Work out the finished part from the listing and answer in its coordinate system (mm). Face numbers are marked on the shaded views. A direction names the side the tool comes from. Give positions to 0.01 mm unless a question says otherwise; leave off trailing zeros. Loops run counter-clockwise (first coordinate to the right, second up) from the corner with the lowest first, then second, coordinate; pieces in that order, holes last. Notation, with made-up numbers: M 88,89.25 L 117,89.25 A18 ccw 117,119.25 Z; hole C -30.75,-39.75 d5. An arc over 180 degrees is marked long. Write item = value, one per line. Start each with the question number.
1. Section B-B on y = 84 is taken. Determine the outline of the cut face in (x, z).
2. Flat-ended cylindrical pins translate along their axes: pin 1 Ø2.5 at (x, z) = (20, 23) entering from -Y; pin 2 Ø2 at (x, z) = (17.5, 16) entering from +Y; pin 3 Ø1 at (x, z) = (4, 9) entering from +Y. Find the tip coordinate at first contact, or state that the pin passes through.
3. For the marked faces 1, 2 and 3, determine the directions among +Z, -Z, +X, -X, +Y, -Y from which every point of the face is accessible in a straight line to the end or side of a thin tool.
4. Section A-A on y = 0 is taken. Determine the outline of the cut face in (x, z) (3 decimals), plus the area to 3 significant figures.
5. Consider L1, parallel to Y at x = 33.35, z = 6; L2, parallel to X at y = -20.5, z = 17.25; L3, parallel to Y at x = 23.5, z = 14.75. Determine where each line is inside the solid, lowest interval first. Write a range as [from, to].
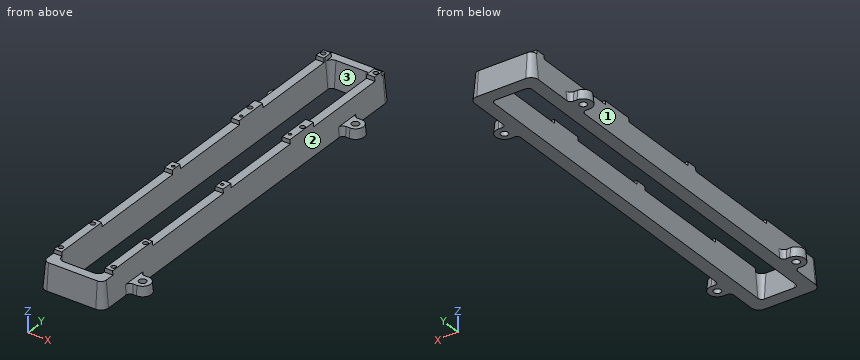
```python
from build123d import *

# Parameters (mm, degrees)
F1_DEPTH      = 25.4
F1_TAPER      = 5
F3_DEPTH      = 304.8010001
F3_DEPTH_BACK = 38.1010001
F4_W          = 70.425
F4_H          = 3.4
F4_W_2        = 84.225
F5_DEPTH      = 40.7760001
F5_DEPTH_BACK = 40.7760001
F6_W          = 73
F6_H          = 3.4
F7_DEPTH      = 40.7760001
F7_DEPTH_BACK = 40.7760001
F9_DEPTH      = 16.0010001
F10_R         = 3.1
F11_DEPTH     = 25.4010001
F12_R         = 2
F12_R_2       = 1.25
F13_DEPTH     = 11


with BuildPart() as f1:
    # F0 (on Top) → F1 (new body)
    with BuildSketch(Plane.XY):
        with BuildLine():
            Line((20.65, 304.8), (-20.65, 304.8))
            ThreePointArc((-20.65, 304.8), (-25.1401280605, 302.9401280605), (-27, 298.45))
            Line((-27, 298.45), (-27, 264.625))
            ThreePointArc((-27, 264.625), (-27.9372583002, 262.3622583002), (-30.2, 261.425))
            Line((-30.2, 261.425), (-33.35, 261.425))
            ThreePointArc((-33.35, 261.425), (-40.775, 254), (-33.35, 246.575))
            Line((-33.35, 246.575), (-30.2, 246.575))
            ThreePointArc((-30.2, 246.575), (-27.9372583002, 245.6377416998), (-27, 243.375))
            Line((-27, 243.375), (-27, 10.625))
            ThreePointArc((-27, 10.625), (-27.9372583002, 8.3622583002), (-30.2, 7.425))
            Line((-30.2, 7.425), (-33.35, 7.425))
            ThreePointArc((-33.35, 7.425), (-40.775, 0), (-33.35, -7.425))
            Line((-33.35, -7.425), (-30.2, -7.425))
            ThreePointArc((-30.2, -7.425), (-27.9372583002, -8.3622583002), (-27, -10.625))
            Line((-27, -10.625), (-27, -31.75))
            ThreePointArc((-27, -31.75), (-25.1401280605, -36.2401280605), (-20.65, -38.1))
            Line((-20.65, -38.1), (20.65, -38.1))
            ThreePointArc((20.65, -38.1), (25.1401280605, -36.2401280605), (27, -31.75))
            Line((27, -31.75), (27, -10.625))
            ThreePointArc((27, -10.625), (27.9372583002, -8.3622583002), (30.2, -7.425))
            Line((30.2, -7.425), (33.35, -7.425))
            ThreePointArc((33.35, -7.425), (40.775, 0), (33.35, 7.425))
            Line((33.35, 7.425), (30.2, 7.425))
            ThreePointArc((30.2, 7.425), (27.9372583002, 8.3622583002), (27, 10.625))
            Line((27, 10.625), (27, 243.375))
            ThreePointArc((27, 243.375), (27.9372583002, 245.6377416998), (30.2, 246.575))
            Line((30.2, 246.575), (33.35, 246.575))
            ThreePointArc((33.35, 246.575), (40.775, 254), (33.35, 261.425))
            Line((33.35, 261.425), (30.2, 261.425))
            ThreePointArc((30.2, 261.425), (27.9372583002, 262.3622583002), (27, 264.625))
            Line((27, 264.625), (27, 298.45))
            ThreePointArc((27, 298.45), (25.1401280605, 302.9401280605), (20.65, 304.8))
        make_face()
        with BuildLine():
            ThreePointArc((-16, 290.6), (-15.0627416998, 292.8627416998), (-12.8, 293.8))
            Line((-12.8, 293.8), (12.8, 293.8))
            ThreePointArc((12.8, 293.8), (15.0627416998, 292.8627416998), (16, 290.6))
            Line((16, 290.6), (16, -23.9))
            ThreePointArc((16, -23.9), (15.0627416998, -26.1627416998), (12.8, -27.1))
            Line((12.8, -27.1), (-12.8, -27.1))
            ThreePointArc((-12.8, -27.1), (-15.0627416998, -26.1627416998), (-16, -23.9))
            Line((-16, -23.9), (-16, 290.6))
        make_face(mode=Mode.SUBTRACT)
    extrude(amount=F1_DEPTH, taper=F1_TAPER)

    # F2 (on Front) → F3 (cut, two sides)
    with BuildSketch(Plane.XZ) as f3_sk:
        Polygon((-26.2913418254, 8.1), (-24.7777879464, 25.4), (-38.5527879464, 25.4), (-40.0663418254, 8.1), align=None)
        Polygon((38.5527879464, 25.4), (24.7777879464, 25.4), (26.2913418254, 8.1), (40.0663418254, 8.1), align=None)
    extrude(amount=-F3_DEPTH, mode=Mode.SUBTRACT)
    extrude(f3_sk.sketch, amount=F3_DEPTH_BACK, mode=Mode.SUBTRACT)

    # F4 (on Right) → F5 (cut, two sides)
    with BuildSketch(Plane.YZ) as f5_sk:
        with Locations((152.5875, 23.7)):
            Rectangle(F4_W, F4_H)
        Polygon((-23.8, 22), (-23.8, 25.4), (-35.8777879464, 25.4), (-36.1752494024, 22), align=None)
        with Locations((65.9125, 23.7)):
            Rectangle(F4_W_2, F4_H)
    extrude(amount=-F5_DEPTH, mode=Mode.SUBTRACT)
    extrude(f5_sk.sketch, amount=F5_DEPTH_BACK, mode=Mode.SUBTRACT)

    # F6 (on Right) → F7 (cut, two sides)
    with BuildSketch(Plane.YZ) as f7_sk:
        Polygon((302.8752494024, 22), (302.5777879464, 25.4), (297.5, 25.4), (297.5, 22), align=None)
        with Locations((252.3, 23.7)):
            Rectangle(F6_W, F6_H)
    extrude(amount=-F7_DEPTH, mode=Mode.SUBTRACT)
    extrude(f7_sk.sketch, amount=F7_DEPTH_BACK, mode=Mode.SUBTRACT)

    # F8 (on face) → F9 (cut, through all)
    with BuildSketch(Plane.XZ.offset(-288.8)):
        Polygon((-18.2222120536, 25.4), (-17.9247505976, 22), (17.9247505976, 22), (18.2222120536, 25.4), align=None)
    extrude(amount=-F9_DEPTH, mode=Mode.SUBTRACT)

    # F10 (on face) → F11 (cut, through all)
    with BuildSketch(Plane(origin=(0, 0, 0), x_dir=(1, 0, 0), z_dir=(0, 0, -1))):
        with Locations((-33.35, 0)):
            Circle(F10_R)
        with Locations((33.35, 0)):
            Circle(F10_R)
        with Locations((-33.35, -254)):
            Circle(F10_R)
        with Locations((33.35, -254)):
            Circle(F10_R)
    extrude(amount=-F11_DEPTH, mode=Mode.SUBTRACT)

    # F12 (on face) → F13 (cut)
    with BuildSketch(Plane.XY.offset(25.4)):
        with Locations((22.225, -19.05)):
            Circle(F12_R)
        with Locations((22.225, 19.05)):
            Circle(F12_R)
        with Locations((-22.225, 19.05)):
            Circle(F12_R)
        with Locations((-22.225, -19.05)):
            Circle(F12_R)
        with Locations((22.225, 293.7)):
            Circle(F12_R)
        with Locations((22.225, 206.4)):
            Circle(F12_R)
        with Locations((-22.225, 206.4)):
            Circle(F12_R)
        with Locations((-22.225, 293.7)):
            Circle(F12_R)
        with Locations((20.65, 193.66)):
            Circle(F12_R_2)
        with Locations((20.65, 112.7)):
            Circle(F12_R_2)
        with Locations((-20.65, 112.7)):
            Circle(F12_R_2)
        with Locations((-20.65, 193.66)):
            Circle(F12_R_2)
    extrude(amount=-F13_DEPTH, mode=Mode.SUBTRACT)


solid = f1.part
```
Verdict:
q1.outline = M -27,0 L -16,0 L -17.92,22 L -25.08,22 Z; M 16,0 L 27,0 L 25.08,22 L 17.92,22 Z
q2.pin_1 = -36.2
q2.pin_2 = 303.49
q2.pin_3 = 304.06
q3.face_1 = +Z, -X
q3.face_2 = +Z, +X
q3.face_3 = +Z
q4.outline = M -40.775,0 L -36.45,0 L -36.45,8.1 L -40.066,8.1 Z; M -30.25,0 L -16,0 L -18.222,25.4 L -24.778,25.4 L -26.291,8.1 L -30.25,8.1 Z; M 16,0 L 30.25,0 L 30.25,8.1 L 26.291,8.1 L 24.778,25.4 L 18.222,25.4 Z; M 36.45,0 L 40.775,0 L 40.066,8.1 L 36.45,8.1 Z
q4.area = 569 mm2
q5.L1 = [-6.9, -3.1], [3.1, 6.9], [247.1, 250.9], [257.1, 260.9]
q5.L2 = [-25.49, -23.6], [-20.85, -17.51], [17.51, 20.85], [23.6, 25.49]
q5.L3 = [-35.93, -20.59], [-17.51, 17.51], [20.59, 204.86], [207.94, 292.16], [295.24, 302.63]
